For this review, take the finished solid that the model builds, in its own axes (mm). A direction names the side the tool comes from. Give positions to 0.01 mm unless a question says otherwise; leave off trailing zeros. Order: outer loops, then holes, each group sorted by start corner. A loop starts at its lowest first (then second) coordinate and runs counter-clockwise, first axis right, second up.
Autodesk Inventor part; units mm, degrees
ref_plane "YZ Plane" through (0, 0, 0) normal (1, 0, 0) x (0, 1, 0)
ref_plane "XZ Plane" through (0, 0, 0) normal (0, 1, 0) x (-1, 0, 0)
ref_plane "XY Plane" through (0, 0, 0) normal (0, 0, 1) x (1, 0, 0)
sketch "Sketch1" plane through (0, 0, 0) normal (0, 1, 0) x (-1, 0, 0)
  line L0 (10, 25) -> (-10, 25)
  line L1 (-10, 25) -> (-10, -25)
  line L2 (-10, -25) -> (10, -25)
  line L3 (10, -25) -> (10, 25)
  line L4 (10, 25) -> (-10, -25) construction
  line L5 (-10, 25) -> (10, -25) construction
  line L6 (0, 0) -> (0, -18)
  line L7 (0, -18) -> (0, 18)
  line L8 (0, 18) -> (2, 18)
  line L9 (0, -18) -> (2, -18)
  circle A0 centre (2, 18) radius 1.5
  circle A1 centre (2, -18) radius 1.5
  dimension "d0" = 20
  dimension "d1" = 50
  dimension "d2" = 18
  dimension "d3" = 36
  dimension "d4" = 2
  dimension "d5" = 2
  dimension "d6" = 3
  dimension "d7" = 3
extrude "Extrusion1" add sketch "Sketch1" against normal blind 2
sketch "Sketch2" plane through (0, 0, 0) normal (0, 1, 0) x (1, 0, 0)
  line L0 (10, 25) -> (10, -25)
  line L1 (10, -25) -> (7, -25)
  line L2 (10, -25) -> (-10, -25)
  line L3 (7, -25) -> (7, 25)
  line L4 (-10, 25) -> (10, 25)
  line L5 (7, 25) -> (10, 25)
  line L6 (10, 25) -> (10, -25)
  point P0 (0, 0)
  dimension "d10" = 3
extrude "Extrusion2" add sketch "Sketch2" along normal blind 10
sketch "Sketch3" plane through (10, -2, 25) normal (1, 0, 0) x (0, 0, -1)
  line L0 (50, 0) -> (0, 0)
  line L1 (25, 0) -> (25, 6)
  line L2 (25, 6) -> (45, 6)
  line L3 (45, 6) -> (25, 6)
  line L4 (25, 6) -> (5, 6)
  line L5 (5, 6) -> (10, 6)
  line L6 (10, 6) -> (40, 6)
  circle A0 centre (40, 6) radius 1.5
  circle A1 centre (10, 6) radius 1.5
  point P0 (25, 2)
  dimension "d13" = 6
  dimension "d14" = 20
  dimension "d15" = 20
  dimension "d16" = 20
  dimension "d17" = 5
  dimension "d18" = 30
  dimension "d19" = 3
  dimension "d20" = 3
extrude "Extrusion3" cut sketch "Sketch3" against normal blind 10
fillet "Fillet1" radius 2 1 edges at (7, 0, 0)
properties part number "IR_holder" material "Aluminum, Anodized Red"
1) Clearance check with flat-ended pins moving along their axes: pin 1 (5 mm diameter, centred on y = 4, z = 15, fed in from -X); pin 2 (4 mm diameter, centred on y = 5, z = 14.5, fed in from +X); pin 3 (4 mm diameter, centred on y = 5.5, z = -4, fed in from -X); pin 4 (7.5 mm diameter, centred on x = 1, z = 4.5, fed in from +Y). State where each tip first meets the part, or that it passes through.
Answer sheet:
pin 1: stops at x = 6.94
pin 2: stops at x = 10
pin 3: stops at x = 7
pin 4: stops at y = 0
2) Tool access review of faces 1 (the face through (7, 6, 0)), 2 (the face through (4.5, -0.4, -25)): name each direction out of +Z, -Z, +X, -X, +Y, -Y from which nothing blocks a thin tool from reaching the whole face with its end or side.
Answer sheet:
face 1: +Z, -Z, -X, +Y
face 2: -Z, +X, -X, +Y, -Y
3) We need section A-A on y = 4. Give the boundary of the cut face in (x, z).
Answer sheet:
outline: (7, -25) - (10, -25) - (10, -16.5) - (7, -16.5) - close; (7, -13.5) - (10, -13.5) - (10, 13.5) - (7, 13.5) - close; (7, 16.5) - (10, 16.5) - (10, 25) - (7, 25) - close
4) We need section D-D on z = 20. Give the boundary of the cut face in (x, y).
Answer sheet:
outline: (-10, -2) - (10, -2) - (10, 10) - (7, 10) - (7, 2) arc R2 cw to (5, 0) - (-10, 0) - close
5) We need section B-B on x = -2. Give the boundary of the cut face in (y, z).
Answer sheet:
outline: (-2, -25) - (0, -25) - (0, -19.5) - (-2, -19.5) - close; (-2, -16.5) - (0, -16.5) - (0, 16.5) - (-2, 16.5) - close; (-2, 19.5) - (0, 19.5) - (0, 25) - (-2, 25) - close
6) To check wall thickness, follow line 1 (Z direction, x = -2, y = -0.4); line 2 (Z direction, x = 9.2, y = 4); line 3 (Y direction, x = 8.5, z = 15). State the ranges of each line that lie inside material, in increasing order.
Answer sheet:
line 1: z = -25 to -19.5, -16.5 to 16.5, 19.5 to 25
line 2: z = -25 to -16.5, -13.5 to 13.5, 16.5 to 25
line 3: y = -2 to 2.5, 5.5 to 10
7) Draft analysis for pull direction Y (two halves, no side actions). For faces 3 (the face through (-2, 0, 0)), 4 (the face through (8.52, 4.07, -13.5)), 5 (the face through (-0.89, -0.99, -16.99)), 6 (the face through (8.52, 4.07, 16.5)), state which applies: +Y half, -Y half, draft (parallel to the pull), parting line (faces both ways), or undercut.
Answer sheet:
face 3: +Y half
face 4: undercut
face 5: draft
face 6: undercut
8) We need section C-C on z = -15. Give the boundary of the cut face in (x, y).
Answer sheet:
outline: (-10, -2) - (10, -2) - (10, 2.5) - (7, 2.5) - (7, 2) arc R2 cw to (5, 0) - (-10, 0) - close; (7, 5.5) - (10, 5.5) - (10, 10) - (7, 10) - close
